Design review of the part built by this model. Coordinates are the model's own, in mm. A direction names the side the tool comes from. Coordinates: 2 decimals unless noted, no trailing zeros. Write each loop counter-clockwise with the first axis right and the second up, starting at its lowest first coordinate (ties: lowest second). Pieces come first, ordered by that corner, then holes.
Q1. For pin 1 Ø5.5 at (x, y) = (-42, -5) entering from +Z; pin 2 Ø5 at (x, y) = (-33, 41) entering from -Z, all flat-tipped, find the tip position at first contact; note any pin that passes through.
Q2. The part is to be moulded in two halves that separate along Y. For faces 3 (the flat face through (-1, 1, 12)), 4 (the flat face through (-1, -47, 6)), 5 (the flat face through (-38.6, 4.6, 6)), say which applies: released by +Y, released by -Y, zero draft, split by the parting line, or undercut.
Q3. Take a section at B-B, the plane y = 21. Write out the cut boundary in (x, z), plus the area to 3 significant figures.
Q4. For faces 1 (the cylindrical face through (7.284, -35.547, 9.042)), 2 (the flat face through (0, 29.5, 6)), list the 3-axis set-ups (+Z, -Z, +X, -X, +Y, -Y) from which the entire face can be reached by the end or side of a thin tool; tool diameter is ignored.
Q5. Take a section at D-D, the plane z = 3. State how many separate pieces and enclosed holes the cut face has, plus the area to 3 significant figures.
Q6. Take a section at C-C, the plane x = -33. Write out the cut boundary in (y, z), plus the area to 3 significant figures.
Q7. Take a section at A-A, the plane x = -22.5. Write out the cut boundary in (y, z).
Q8. For L1, parallel to Y at x = 33, z = 3.7; L2, parallel to Y at x = 41, z = 2.9; L3, parallel to X at y = -41, z = 2.5, list the stretches that pass through material, from the lowest coordinate up.
from build123d import *

# Parameters (mm, degrees)
SKETCH_1_W          = 94
SKETCH_1_H          = 94
SKETCH_1_R          = 3
SKETCH_1_W_2        = 50
SKETCH_1_H_2        = 12
EXTRUDE_1_DEPTH     = 12
SKETCH_2_R          = 5.5
CUT_EXTRUDE_1_DEPTH = 6


with BuildPart() as part:
    # 草图1 → 凸台-拉伸1 (new body)
    with BuildSketch(Plane.XY):
        Rectangle(SKETCH_1_W, SKETCH_1_H)
        with Locations((-33, 41)):
            Circle(SKETCH_1_R, mode=Mode.SUBTRACT)
        with Locations((-8, 41)):
            Circle(SKETCH_1_R, mode=Mode.SUBTRACT)
        with Locations((-41, 21)):
            Circle(SKETCH_1_R, mode=Mode.SUBTRACT)
        with Locations((-41, 7)):
            Circle(SKETCH_1_R, mode=Mode.SUBTRACT)
        with Locations((-41, -7)):
            Circle(SKETCH_1_R, mode=Mode.SUBTRACT)
        with Locations((-41, -21)):
            Circle(SKETCH_1_R, mode=Mode.SUBTRACT)
        with Locations(Location((-8, -41, 0), (0, 0, 180))):
            Circle(SKETCH_1_R, mode=Mode.SUBTRACT)
        with Locations(Location((-33, -41, 0), (0, 0, 180))):
            Circle(SKETCH_1_R, mode=Mode.SUBTRACT)
        with Locations((33, -41)):
            Circle(SKETCH_1_R, mode=Mode.SUBTRACT)
        with Locations((8, -41)):
            Circle(SKETCH_1_R, mode=Mode.SUBTRACT)
        with Locations(Location((41, -21, 0), (0, 0, 180))):
            Circle(SKETCH_1_R, mode=Mode.SUBTRACT)
        with Locations(Location((41, -7, 0), (0, 0, 180))):
            Circle(SKETCH_1_R, mode=Mode.SUBTRACT)
        with Locations(Location((41, 7, 0), (0, 0, 180))):
            Circle(SKETCH_1_R, mode=Mode.SUBTRACT)
        with Locations(Location((41, 21, 0), (0, 0, 180))):
            Circle(SKETCH_1_R, mode=Mode.SUBTRACT)
        with Locations(Location((8, 41, 0), (0, 0, 180))):
            Circle(SKETCH_1_R, mode=Mode.SUBTRACT)
        with Locations(Location((33, 41, 0), (0, 0, 180))):
            Circle(SKETCH_1_R, mode=Mode.SUBTRACT)
        with Locations((-9, 11.5)):
            Circle(SKETCH_1_R, mode=Mode.SUBTRACT)
        with Locations((9, 11.5)):
            Circle(SKETCH_1_R, mode=Mode.SUBTRACT)
        with Locations((0, 23.5)):
            Rectangle(SKETCH_1_W_2, SKETCH_1_H_2, mode=Mode.SUBTRACT)
    extrude(amount=EXTRUDE_1_DEPTH)

    # 草图2 → 切除-拉伸1 (cut)
    with BuildSketch(Plane.XY.offset(12)):
        with Locations((-33, 41)):
            Circle(SKETCH_2_R)
        with Locations((-8, 41)):
            Circle(SKETCH_2_R)
        with Locations((-41, 21)):
            Circle(SKETCH_2_R)
        with Locations(Location((41, 7, 0), (0, 0, 180))):
            Circle(SKETCH_2_R)
        with Locations((-41, 7)):
            Circle(SKETCH_2_R)
        with Locations(Location((41, 21, 0), (0, 0, 180))):
            Circle(SKETCH_2_R)
        with Locations(Location((8, 41, 0), (0, 0, 180))):
            Circle(SKETCH_2_R)
        with Locations(Location((33, 41, 0), (0, 0, 180))):
            Circle(SKETCH_2_R)
        with Locations((33, -41)):
            Circle(SKETCH_2_R)
        with Locations((8, -41)):
            Circle(SKETCH_2_R)
        with Locations((41, -21)):
            Circle(SKETCH_2_R)
        with Locations(Location((-41, -7, 0), (0, 0, 180))):
            Circle(SKETCH_2_R)
        with Locations((41, -7)):
            Circle(SKETCH_2_R)
        with Locations(Location((-41, -21, 0), (0, 0, 180))):
            Circle(SKETCH_2_R)
        with Locations(Location((-8, -41, 0), (0, 0, 180))):
            Circle(SKETCH_2_R)
        with Locations(Location((-33, -41, 0), (0, 0, 180))):
            Circle(SKETCH_2_R)
    extrude(amount=-CUT_EXTRUDE_1_DEPTH, mode=Mode.SUBTRACT)


solid = part.part
Responses:
1. pin 1: stops at z = 6
1. pin 2: passes through
2. face 3: zero draft
2. face 4: released by -Y
2. face 5: undercut
3. outline: (-47, 0) - (-44, 0) - (-44, 6) - (-46.5, 6) - (-46.5, 12) - (-47, 12) - close; (-38, 0) - (-25, 0) - (-25, 12) - (-35.5, 12) - (-35.5, 6) - (-38, 6) - close; (25, 0) - (38, 0) - (38, 6) - (35.5, 6) - (35.5, 12) - (25, 12) - close; (44, 0) - (47, 0) - (47, 12) - (46.5, 12) - (46.5, 6) - (44, 6) - close
3. area: 324 mm2
4. face 1: +Z
4. face 2: +Z, -Z
5. separate pieces: 1
5. enclosed holes: 19
5. area: 7,730 mm2
6. outline: (-47, 0) - (-44, 0) - (-44, 6) - (-46.5, 6) - (-46.5, 12) - (-47, 12) - close; (-38, 0) - (38, 0) - (38, 6) - (35.5, 6) - (35.5, 12) - (-35.5, 12) - (-35.5, 6) - (-38, 6) - close; (44, 0) - (47, 0) - (47, 12) - (46.5, 12) - (46.5, 6) - (44, 6) - close
6. area: 924 mm2
7. outline: (-47, 0) - (17.5, 0) - (17.5, 12) - (-47, 12) - close; (29.5, 0) - (47, 0) - (47, 12) - (29.5, 12) - close
8. L1: y = -47 to -44, -38 to 38, 44 to 47
8. L2: y = -47 to -24, -18 to -10, -4 to 4, 10 to 18, 24 to 47
8. L3: x = -47 to -36, -30 to -11, -5 to 5, 11 to 30, 36 to 47
